Can you work these out from the model? Positions are in its coordinate system, mm. Coordinates: 2 decimals unless noted, no trailing zeros. Order: outer loops, then holes, each group sorted by start corner. A loop starts at its lowest first (then second) coordinate and runs counter-clockwise, first axis right, second up. Notation, with made-up numbers: M -25.75,86.5 L -19.75,86.5 A16 ccw -19.75,107.5 Z; hole C 1.25,26 d9. An arc over 180 degrees is marked long. Answer as a JSON object with one key per item and string values.
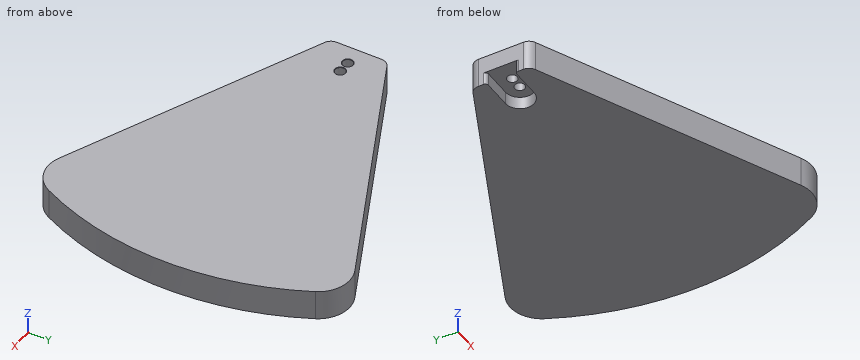
from build123d import *

# Parameters (mm, degrees)
BOSS_EXTRUDE1_DEPTH            = 9.525
CUT_EXTRUDE2_DEPTH             = 4
M3_CLEARANCE_HOLE1_D           = 3.2
M3_CLEARANCE_HOLE1_CSINK_D     = 3.45
M3_CLEARANCE_HOLE1_CSINK_ANGLE = 90
FILLET1_R                      = 1
FILLET2_R                      = 3
FILLET3_R                      = 10


with BuildPart() as part:
    # Sketch2 → Boss-Extrude1 (new body)
    with BuildSketch(Plane(origin=(0, 0, 0), x_dir=(0, 1, 0), z_dir=(0, 0, 1))):
        with BuildLine():
            Line((-9, 10), (9, 10))
            Line((9, 10), (50.45475081, -78.9))
            ThreePointArc((50.45475081, -78.9), (0, -93.653039883), (-50.45475081, -78.9))
            Line((-50.45475081, -78.9), (-9, 10))
        make_face()
    extrude(amount=BOSS_EXTRUDE1_DEPTH)

    # Sketch3 → Cut-Extrude2 (cut)
    with BuildSketch(Plane(origin=(0, 0, 0), x_dir=(1, 0, 0), z_dir=(0, 0, -1))):
        with BuildLine():
            Line((-10, -4.5), (-10, 4.5))
            Line((-10, 4.5), (0, 4.5))
            ThreePointArc((0, 4.5), (4.5, 0), (0, -4.5))
            Line((0, -4.5), (-10, -4.5))
        make_face()
    extrude(amount=-CUT_EXTRUDE2_DEPTH, mode=Mode.SUBTRACT)

    # M3 Clearance Hole1 (through all)
    with Locations(Plane(origin=(0, 0, 9.525), x_dir=(0, -1, 0), z_dir=(0, 0, 1))):
        with Locations((0, 0), (0, -4)):
            CounterSinkHole(M3_CLEARANCE_HOLE1_D / 2, M3_CLEARANCE_HOLE1_CSINK_D / 2, counter_sink_angle=M3_CLEARANCE_HOLE1_CSINK_ANGLE)

    # Fillet1
    fillet1_edges = [part.edges().sort_by_distance(p)[0] for p in [
        (-10, 4.5, 2),
        (-10, -4.5, 2),
    ]]
    fillet(fillet1_edges, radius=FILLET1_R)

    # Fillet2
    fillet2_edges = [part.edges().sort_by_distance(p)[0] for p in [
        (-10, -9, 4.7625),
        (-10, 9, 4.7625),
    ]]
    fillet(fillet2_edges, radius=FILLET2_R)

    # Fillet3
    fillet3_edges = [part.edges().sort_by_distance(p)[0] for p in [
        (78.9, 50.45475081, 4.7625),
        (78.9, -50.45475081, 4.7625),
    ]]
    fillet(fillet3_edges, radius=FILLET3_R)


solid = part.part
Item 1: I want a section at B-B, the plane z = 7. Write out the boundary of the cut face in (x, y).
Answers follow:
{"outline": "M -10,-7.09 A3 ccw -8.27,-9.81 L 70.55,-46.56 A10 ccw 83.72,-41.98 A93.65 ccw 83.72,41.98 A10 ccw 70.55,46.56 L -8.27,9.81 A3 ccw -10,7.09 Z; hole C -4,0 d3.2; hole C 0,0 d3.2"}
Item 2: I want a section at A-A, the plane y = 0. Write out the boundary of the cut face in (x, z) (3 decimals).
Answers follow:
{"outline": "M -10,4 L -5.6,4 L -5.6,9.4 L -5.725,9.525 L -10,9.525 Z; M -2.4,4 L -1.6,4 L -1.6,9.4 L -1.725,9.525 L -2.275,9.525 L -2.4,9.4 Z; M 1.6,4 L 4.5,4 L 4.5,0 L 93.653,0 L 93.653,9.525 L 1.725,9.525 L 1.6,9.4 Z"}
Item 3: Please list where these lines run through material, in increasing order: line 1 (X direction, y = 0, z = 7.35); line 2 (Y direction, x = -5, z = 7.75); line 3 (Y direction, x = 0, z = 8.3).
Answers follow:
{"line 1": "x = -10 to -5.6, -2.4 to -1.6, 1.6 to 93.65", "line 2": "y = -11.33 to -1.25, 1.25 to 11.33", "line 3": "y = -13.66 to -1.6, 1.6 to 13.66"}
Item 4: I'm going to push flat-ended pins straight in: pin 1 (2 mm diameter, centred on x = -3, z = 2, fed in from -Y); pin 2 (3 mm diameter, centred on x = 0, y = 0, fed in from +Z); pin 3 (3 mm diameter, centred on y = 0.5, z = 4.5, fed in from +X); pin 4 (3.5 mm diameter, centred on x = -5, y = 0, fed in from -Z). Where does each tip first touch, or does it pass through?
Answers follow:
{"pin 1": "stops at y = -12.73", "pin 2": "passes through", "pin 3": "stops at x = 93.65", "pin 4": "stops at z = 4"}
Item 5: I want a section at C-C, the plane x = -4. Write out the boundary of the cut face in (y, z) (3 decimals).
Answers follow:
{"outline": "M -11.798,0 L -4.5,0 L -4.5,4 L -1.6,4 L -1.6,9.4 L -1.725,9.525 L -11.798,9.525 Z; M 1.6,4 L 4.5,4 L 4.5,0 L 11.798,0 L 11.798,9.525 L 1.725,9.525 L 1.6,9.4 Z"}
Item 6: I want a section at D-D, the plane x = 31. Write out the boundary of the cut face in (y, z) (3 decimals), plus the area to 3 significant figures.
Answers follow:
{"outline": "M -28.119,0 L 28.119,0 L 28.119,9.525 L -28.119,9.525 Z", "area": "536 mm^2"}
